Geometry check sheet. Reference: the model listing, model coordinates, mm. Face numbers are marked on the shaded views. A direction names the side the tool comes from. Round coordinates to 2 decimals unless told otherwise and drop trailing zeros. Write each loop counter-clockwise with the first axis right and the second up, starting at its lowest first coordinate (ties: lowest second). Pieces come first, ordered by that corner, then holes. Notation, with made-up numbers: M 8.25,3.5 L 58.25,3.5 A27 ccw 58.25,41.5 Z; hole C 44,3.5 d10. An arc over 180 degrees is marked long. Answer in a Markdown table with one row per item. Add a question column.
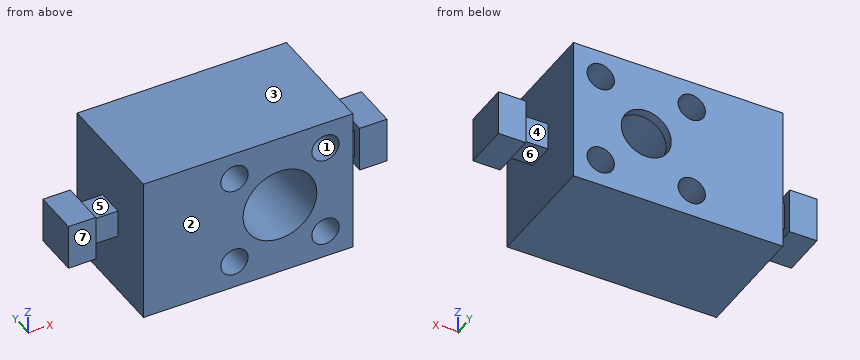
Autodesk Inventor part; units mm, degrees
ref_plane "YZ Plane" through (0, 0, 0) normal (1, 0, 0) x (0, 1, 0)
ref_plane "XZ Plane" through (0, 0, 0) normal (0, 1, 0) x (-1, 0, 0)
ref_plane "XY Plane" through (0, 0, 0) normal (0, 0, 1) x (1, 0, 0)
sketch "Esquisse1" plane through (0, 0, 0) normal (0, 1, 0) x (-1, 0, 0)
  line L0 (4.4286, 5.3714) -> (-11.5714, 5.3714)
  line L1 (-11.5714, 5.3714) -> (-11.5714, -10.6286)
  line L2 (-11.5714, -10.6286) -> (4.4286, -10.6286)
  line L3 (4.4286, -10.6286) -> (4.4286, 5.3714)
  point P0 (0, 0)
  dimension "d0" = 16
  dimension "d1" = 16
extrude "Extrusion1" add sketch "Esquisse1" along normal blind 13
sketch "Esquisse2" plane through (0, 0, 0) normal (0, -1, 0) x (1, 0, 0)
  circle A0 centre (3.5714, -2.6286) radius 4.05
  line L0 (-4.4286, 5.3714) -> (11.5714, 5.3714)
  line L1 (11.5714, 5.3714) -> (11.5714, -10.6286)
  point P0 (0, 0)
  dimension "d4" = 8
  dimension "d5" = 8
  dimension "d6" = 8.1
extrude "Extrusion2" cut sketch "Esquisse2" against normal blind 12
sketch "Esquisse3" plane through (3.5714, 12, -2.6286) normal (0, -1, 0) x (1, 0, 0)
  circle A0 centre (0, 0) radius 2.75
  line L0 (8, -8) -> (-8, -8)
  line L1 (8, 8) -> (8, -8)
  point P0 (-3.5714, 2.6286)
  dimension "d9" = 5.5
  dimension "d10" = 8
  dimension "d11" = 8
extrude "Extrusion3" cut sketch "Esquisse3" against normal through all
sketch "Esquisse4" plane through (0, 0, 0) normal (0, -1, 0) x (1, 0, 0)
  circle A0 centre (8.5714, 2.3714) radius 1.5
  circle A1 centre (-1.4286, 2.3714) radius 1.5
  circle A2 centre (-1.4286, -7.6286) radius 1.5
  circle A3 centre (8.5714, -7.6286) radius 1.5
  line L0 (-4.4286, -10.6286) -> (-4.4286, 5.3714)
  line L1 (-4.4286, 5.3714) -> (11.5714, 5.3714)
  line L2 (11.5714, 5.3714) -> (11.5714, -10.6286)
  line L3 (11.5714, -10.6286) -> (-4.4286, -10.6286)
  point P0 (0, 0)
  dimension "d14" = 3
  dimension "d15" = 3
  dimension "d16" = 3
  dimension "d17" = 3
  dimension "d19" = 3
  dimension "d20" = 3
  dimension "d21" = 3
  dimension "d22" = 3
  dimension "d23" = 3
  dimension "d24" = 3
  dimension "d25" = 3
  dimension "d26" = 3
extrude "Extrusion4" cut sketch "Esquisse4" against normal through all contours A0 | A1 | A2 | A3
sketch "Esquisse6" plane through (11.5714, 0, 5.3714) normal (1, 0, 0) x (0, 0, -1)
  line L0 (6.5, 8) -> (9.5, 8)
  line L1 (9.5, 8) -> (9.5, 5)
  line L2 (9.5, 5) -> (6.5, 5)
  line L3 (6.5, 5) -> (6.5, 8)
  line L4 (0, 0) -> (0, 13)
  line L5 (0, 13) -> (16, 13)
  point P0 (5.3714, 0)
  dimension "d29" = 3
  dimension "d30" = 3
  dimension "d31" = 6.5
  dimension "d32" = 5
extrude "Extrusion5" add sketch "Esquisse6" along normal blind 3
sketch "Esquisse7" plane through (14.5714, 0, 5.3714) normal (1, 0, 0) x (0, 0, -1)
  line L0 (5.5, 9) -> (10.5, 9)
  line L1 (10.5, 9) -> (10.5, 4)
  line L2 (10.5, 4) -> (5.5, 4)
  line L3 (5.5, 4) -> (5.5, 9)
  line L4 (0, 13) -> (16, 13)
  line L5 (0, 0) -> (0, 13)
  point P0 (5.3714, 0)
  dimension "d35" = 5
  dimension "d36" = 5
  dimension "d37" = 4
  dimension "d38" = 5.5
extrude "Extrusion6" add sketch "Esquisse7" along normal blind 3
sketch "Esquisse8" plane through (-4.4286, 0, -10.6286) normal (-1, 0, 0) x (0, 0, 1)
  line L0 (0, 0) -> (0, 13)
  line L1 (0, 13) -> (16, 13)
  line L2 (16, 13) -> (16, 0)
  line L3 (16, 0) -> (0, 0)
  line L4 (0, 0) -> (0, 13)
  point P0 (10.6286, 0)
extrude "Extrusion7" add sketch "Esquisse8" along normal blind 7
sketch "Esquisse9" plane through (-11.4286, 0, -10.6286) normal (-1, 0, 0) x (0, 0, 1)
  line L0 (9.5, 8) -> (6.5, 8)
  line L1 (6.5, 8) -> (6.5, 5)
  line L2 (6.5, 5) -> (9.5, 5)
  line L3 (9.5, 5) -> (9.5, 8)
  line L4 (16, 0) -> (16, 13)
  line L5 (16, 13) -> (0, 13)
  point P0 (10.6286, 0)
  dimension "d43" = 6.5
  dimension "d44" = 5
  dimension "d45" = 3
  dimension "d46" = 3
extrude "Extrusion8" add sketch "Esquisse9" along normal blind 3
sketch "Esquisse10" plane through (-14.4286, 0, -10.6286) normal (-1, 0, 0) x (0, 0, 1)
  line L0 (10.5, 9) -> (5.5, 9)
  line L1 (5.5, 9) -> (5.5, 4)
  line L2 (5.5, 4) -> (10.5, 4)
  line L3 (10.5, 4) -> (10.5, 9)
  line L4 (16, 0) -> (16, 13)
  line L5 (0, 0) -> (16, 0)
  point P0 (10.6286, 0)
  dimension "d49" = 5.5
  dimension "d50" = 4
  dimension "d51" = 5
  dimension "d52" = 5
extrude "Extrusion9" add sketch "Esquisse10" along normal blind 3
properties part number "capuchon_roulement_8_1mm"
Item 1: Access from +Z, -Z, +X, -X, +Y, -Y to the whole of each face (thin tool, end or side, straight path). Record for the marked faces 4, 5, 6 and 7.
Item 2: Section check C-C, the plane y = 2.5. Record the boundary of the cut face in (x, z).
Item 3: Scan lines: probe 1 along Z at (x, y) = (-1.5, 6.5); probe 2 along X at (y, z) = (8, -8.75); probe 3 along X at (y, z) = (8.75, -6.75). Record each from-to range of solid material in increasing order. Write a range as from..to.
Item 4: Mould release check, pull along Z, two halves, no side actions. Record for the marked faces 1, 2 and 3: +Z half, -Z half, draft (parallel to the pull), parting line (faces both ways), or undercut.
Item 5: Gauge pin test, flat ends, axial feed: pin 1 Ø2.5 at (x, z) = (-16.5, -2.5) entering from -Y; pin 2 Ø0.9 at (x, z) = (16, -1.5) entering from +Y; pin 3 Ø3.5 at (x, y) = (-16, 6.5) entering from +Z. Record the tip position at first contact, or that the pin passes through.
Item 6: Section check A-A, the plane x = -2.5. Record the boundary of the cut face in (y, z).
Item 7: Section check B-B, the plane z = -3.75. Record the boundary of the cut face in (x, y).
Item 8: Section check D-D, the plane z = 3.25. Record the boundary of the cut face in (x, y).
Result sheet:
| question | item | result |
|---|---|---|
| 1 | face 4 | +Z, -Z, +Y |
| 1 | face 5 | +Z, +Y, -Y |
| 1 | face 6 | -Z, +Y, -Y |
| 1 | face 7 | +Z, -Z, -X, -Y |
| 2 | outline | M -11.43,-10.63 L 11.57,-10.63 L 11.57,5.37 L -11.43,5.37 Z; hole C -1.43,-7.63 d3; hole C -1.43,2.37 d3; hole C 3.57,-2.63 d8.1; hole C 8.57,-7.63 d3; hole C 8.57,2.37 d3 |
| 3 | probe 1 | z = -10.63..-9.13, -6.13..0.87, 3.87..5.37 |
| 3 | probe 2 | x = -11.43..-2.42, -0.43..7.58, 9.57..11.57 |
| 3 | probe 3 | x = -11.43..-2.64, -0.21..7.36, 9.79..11.57 |
| 4 | face 1 | undercut |
| 4 | face 2 | draft |
| 4 | face 3 | +Z half |
| 5 | pin 1 | stops at y = 4 |
| 5 | pin 2 | stops at y = 9 |
| 5 | pin 3 | stops at z = -0.13 |
| 6 | outline | M 0,-10.63 L 13,-10.63 L 13,-8.68 L 0,-8.68 Z; M 0,-6.58 L 13,-6.58 L 13,1.32 L 0,1.32 Z; M 0,3.42 L 13,3.42 L 13,5.37 L 0,5.37 Z |
| 7 | outline | M -17.43,4 L -14.43,4 L -14.43,5 L -11.43,5 L -11.43,0 L -0.32,0 L -0.32,12 L 1.06,12 L 1.06,13 L -11.43,13 L -11.43,8 L -14.43,8 L -14.43,9 L -17.43,9 Z; M 6.08,12 L 7.46,12 L 7.46,0 L 11.57,0 L 11.57,5 L 14.57,5 L 14.57,4 L 17.57,4 L 17.57,9 L 14.57,9 L 14.57,8 L 11.57,8 L 11.57,13 L 6.08,13 Z |
| 8 | outline | M -11.43,0 L -2.64,0 L -2.64,13 L -11.43,13 Z; M -0.21,0 L 7.36,0 L 7.36,13 L -0.21,13 Z; M 9.79,0 L 11.57,0 L 11.57,13 L 9.79,13 Z |
